Model file for the job. Use its own axes, mm. Coordinates: 2 decimals unless noted, no trailing zeros. Write each loop counter-clockwise with the first axis right and the second up, starting at its lowest first coordinate (ties: lowest second). Pieces come first, ordered by that corner, then holes. Notation, with made-up numbers: (69, 29.25) - (90, 29.25) arc R19 cw to (90, 52.25) - close; hole circle Ø4 at (50.25, -14.75). An arc over 180 degrees is marked (long way). Put each result on its own line as item: value. Start each with the question number.
1. Drill centre lines: L1, parallel to Y at x = 23, z = 0.85; L2, parallel to Y at x = -39.5, z = 0.4; L3, parallel to X at y = -0.5, z = 0.25. Where is each one in solid material? Low to high. Write a range as from..to.
2. Saw through at A-A, the plane z = 0.95. Write the cut outline in (x, y).
3. Saw through at D-D, the plane y = -23. Write the cut outline in (x, z).
4. Saw through at B-B, the plane y = 0. Write the cut outline in (x, z).
5. Drop flat-ended pins along their axis: P1, Ø1, axis at x = -22, z = 1, coming from the +Y side; P2, Ø1, axis at x = 43, z = 1.5, coming from the -Y side; P3, Ø1, axis at x = 17, z = 1.5, coming from the -Y side. Give the stop position or say it passes through.
6. Saw through at C-C, the plane x = 19.5. Write the cut outline in (y, z).
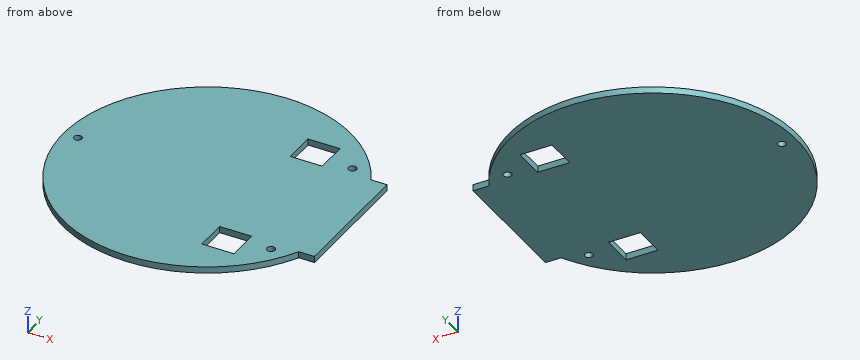
```python
from build123d import *

# Parameters (mm, degrees)
SKETCH1_R  = 1.25
SKETCH1_W  = 10
SKETCH1_H  = 10
BODY_DEPTH = 2


with BuildPart() as part:
    # Sketch1 → Body (new body)
    with BuildSketch(Plane.XY):
        with BuildLine():
            Line((45, 20.5), (40.059330998, 20.5))
            ThreePointArc((40.059330998, 20.5), (-45, 0), (40.059330998, -20.5))
            Line((40.059330998, -20.5), (45, -20.5))
            Line((45, -20.5), (45, 20.5))
        make_face()
        with Locations((-40.427264064, 0)):
            Circle(SKETCH1_R, mode=Mode.SUBTRACT)
        with Locations((32.798809505, -23)):
            Circle(SKETCH1_R, mode=Mode.SUBTRACT)
        with Locations((32.798809505, 23)):
            Circle(SKETCH1_R, mode=Mode.SUBTRACT)
        with Locations((20, 25)):
            Rectangle(SKETCH1_W, SKETCH1_H, mode=Mode.SUBTRACT)
        with Locations((20, -25)):
            Rectangle(SKETCH1_W, SKETCH1_H, mode=Mode.SUBTRACT)
    extrude(amount=BODY_DEPTH)


solid = part.part
```
Final values:
1. L1: y = -38.68..-30, -20..20, 30..38.68
1. L2: y = -21.56..-0.84, 0.84..21.56
1. L3: x = -45..-41.57, -39.28..45
2. outline: (40.06, -20.5) - (45, -20.5) - (45, 20.5) - (40.06, 20.5) arc R45 ccw (long way) to start; hole circle Ø2.5 at (-40.43, 0); hole (15, -30) - (25, -30) - (25, -20) - (15, -20) - close; hole (15, 20) - (25, 20) - (25, 30) - (15, 30) - close; hole circle Ø2.5 at (32.8, -23); hole circle Ø2.5 at (32.8, 23)
3. outline: (-38.68, 0) - (15, 0) - (15, 2) - (-38.68, 2) - close; (25, 0) - (31.55, 0) - (31.55, 2) - (25, 2) - close; (34.05, 0) - (38.68, 0) - (38.68, 2) - (34.05, 2) - close
4. outline: (-45, 0) - (-41.68, 0) - (-41.68, 2) - (-45, 2) - close; (-39.18, 0) - (45, 0) - (45, 2) - (-39.18, 2) - close
5. P1: stops at y = 39.53
5. P2: stops at y = -20.5
5. P3: stops at y = -41.87
6. outline: (-40.56, 0) - (-30, 0) - (-30, 2) - (-40.56, 2) - close; (-20, 0) - (20, 0) - (20, 2) - (-20, 2) - close; (30, 0) - (40.56, 0) - (40.56, 2) - (30, 2) - close
